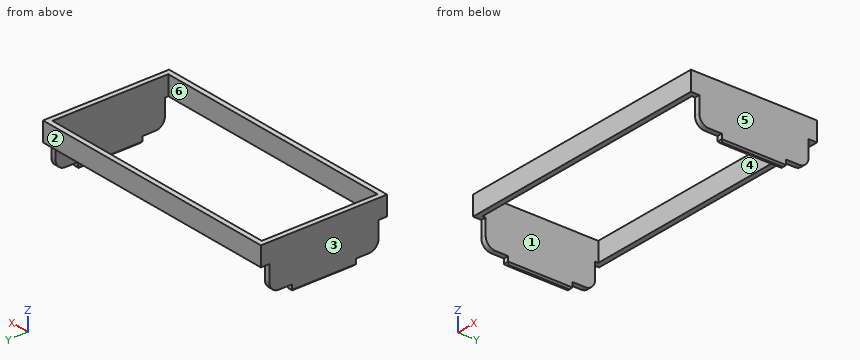
from build123d import *

# Parameters (mm, degrees)
SKETCH1_W           = 80.8
SKETCH1_H           = 39.2
SKETCH1_W_2         = 77.6
SKETCH1_H_2         = 36
BOSS_EXTRUDE1_DEPTH = 6
SKETCH2_W           = 1.6
SKETCH2_H           = 36
BOSS_EXTRUDE2_DEPTH = 8
MOVE_FACE1_BY       = 1
MOVE_FACE1_2_BY     = 1
MOVE_FACE1_3_BY     = 1
MOVE_FACE1_4_BY     = 1
SKETCH3_W           = 1.6
SKETCH3_H           = 20
BOSS_EXTRUDE3_DEPTH = 2
CHAMFER1_SIZE       = 0.5
FILLET1_R           = 3


with BuildPart() as part:
    # Sketch1 → Boss-Extrude1 (new body)
    with BuildSketch(Plane.XY):
        with Locations((38.8, -18)):
            Rectangle(SKETCH1_W, SKETCH1_H)
        with Locations((38.8, -18)):
            Rectangle(SKETCH1_W_2, SKETCH1_H_2, mode=Mode.SUBTRACT)
    extrude(amount=BOSS_EXTRUDE1_DEPTH)

    # Sketch2 → Boss-Extrude2 (add)
    with BuildSketch(Plane(origin=(0, 0, 0), x_dir=(-1, 0, 0), z_dir=(0, 0, -1))):
        with Locations((-78.4, -18)):
            Rectangle(SKETCH2_W, SKETCH2_H)
        with Locations((0.8, -18)):
            Rectangle(SKETCH2_W, SKETCH2_H)
    extrude(amount=BOSS_EXTRUDE2_DEPTH)

    # Move Face1: a face moved inward by 1.0
    extrude(part.faces().sort_by_distance((78.4, 0, -4))[0], amount=MOVE_FACE1_BY, dir=(0, -1, 0), mode=Mode.SUBTRACT)

    # Move Face1 2: a face moved inward by 1.0
    extrude(part.faces().sort_by_distance((78.4, -36, -4))[0], amount=MOVE_FACE1_2_BY, dir=(0, 1, 0), mode=Mode.SUBTRACT)

    # Move Face1 3: a face moved inward by 1.0
    extrude(part.faces().sort_by_distance((-0.8, -36, -4))[0], amount=MOVE_FACE1_3_BY, dir=(0, 1, 0), mode=Mode.SUBTRACT)

    # Move Face1 4: a face moved inward by 1.0
    extrude(part.faces().sort_by_distance((-0.8, 0, -4))[0], amount=MOVE_FACE1_4_BY, dir=(0, -1, 0), mode=Mode.SUBTRACT)

    # Sketch3 → Boss-Extrude3 (add)
    with BuildSketch(Plane(origin=(0, 0, -8), x_dir=(-1, 0, 0), z_dir=(0, 0, -1))):
        with Locations((-78.4, -18)):
            Rectangle(SKETCH3_W, SKETCH3_H)
        with Locations((0.8, -18)):
            Rectangle(SKETCH3_W, SKETCH3_H)
    extrude(amount=BOSS_EXTRUDE3_DEPTH)

    # Chamfer1
    chamfer1_edges = [part.edges().sort_by_distance(p)[0] for p in [
        (78.4, -28, -10),
        (77.6, -18, -10),
        (78.4, -8, -10),
        (79.2, -18, -10),
        (0, -18, -10),
        (-0.8, -28, -10),
        (-1.6, -18, -10),
        (-0.8, -8, -10),
    ]]
    chamfer(chamfer1_edges, length=CHAMFER1_SIZE)

    # Fillet1
    fillet1_edges = [part.edges().sort_by_distance(p)[0] for p in [
        (78.4, -1, -8),
        (78.4, -35, -8),
        (-0.8, -1, -8),
        (-0.8, -35, -8),
    ]]
    fillet(fillet1_edges, radius=FILLET1_R)


solid = part.part
Could you check a few things on this model? Use its own coordinates, in mm. Face numbers are marked on the shaded views. A direction names the side the tool comes from. Give positions to 0.01 mm unless a question says otherwise; leave off trailing zeros. Write each loop counter-clockwise with the first axis right and the second up, starting at its lowest first coordinate (ties: lowest second). Pieces come first, ordered by that corner, then holes. Notation, with made-up numbers: (60, 54) - (79, 54) arc R30 ccw to (79, 81) - close; hole circle Ø2 at (-29.5, -36.75). An arc over 180 degrees is marked (long way). Use CSV: the item, a comma, the result in double quotes. Start each with the question number.
Item 1: For the marked faces 5 and 6, which set-ups out of +Z, -Z, +X, -X, +Y, -Y let a thin tool reach every point of the face, with its end or its side?
Item 2: I want a section at C-C, the plane z = 3.25. Please give me the cut outline in (x, y), then the cut area to 3 significant figures.
Item 3: If we mould it in two halves opening along Y, with no side actions, what happens to the marked faces 1, 2, 3 and 4? For each: pulls with the +Y half, pulls with the -Y half, needs draft (parallel to the pull), parting line crosses it, or undercut.
Item 4: I'm going to push flat-ended pins straight in: pin 1 (6 mm diameter, centred on x = 37.5, z = -4, fed in from -Y); pin 2 (1.3 mm diameter, centred on x = -0.5, z = -2, fed in from -Y); pin 3 (1.3 mm diameter, centred on x = -1, y = -30.5, fed in from -Z); pin 4 (1.6 mm diameter, centred on x = -0.5, z = -8.5, fed in from +Y). Where does each tip first touch, or does it pass through?
Item 5: I want a section at A-A, the plane y = -5.5. Please give me the cut outline in (x, z), then the cut area to 3 significant figures.
Item 6: If I drill on line 1 along X through (y, z) = (-17, -8); line 2 along Y through (x, z) = (15.5, 3.75), over which ranges is the centre line in solid material (lowest first)?
Item 7: I want a section at B-B, the plane z = -1.5. Please give me the cut outline in (x, y), then the cut area to 3 significant figures.
Item 8: I want a section at D-D, the plane y = -20. Please give me the cut outline in (x, z).
Findings:
1,face 5,"+Z, -Z, +X, +Y, -Y"
1,face 6,"+Z, -Z"
2,outline,"(-1.6, -37.6) - (79.2, -37.6) - (79.2, 1.6) - (-1.6, 1.6) - close; hole (0, -36) - (77.6, -36) - (77.6, 0) - (0, 0) - close"
2,area,"374 mm2"
3,face 1,"undercut"
3,face 2,"pulls with the +Y half"
3,face 3,"needs draft"
3,face 4,"undercut"
4,pin 1,"passes through"
4,pin 2,"stops at y = -35"
4,pin 3,"stops at z = -8"
4,pin 4,"stops at y = -2.69"
5,outline,"(-1.6, -8) - (0, -8) - (0, 6) - (-1.6, 6) - close; (77.6, -8) - (79.2, -8) - (79.2, 6) - (77.6, 6) - close"
5,area,"44.8 mm2"
6,line 1,"x = -1.6 to 0, 77.6 to 79.2"
6,line 2,"y = -37.6 to -36, 0 to 1.6"
7,outline,"(-1.6, -35) - (0, -35) - (0, -1) - (-1.6, -1) - close; (77.6, -35) - (79.2, -35) - (79.2, -1) - (77.6, -1) - close"
7,area,"109 mm2"
8,outline,"(-1.6, -9.5) - (-1.1, -10) - (-0.5, -10) - (0, -9.5) - (0, 6) - (-1.6, 6) - close; (77.6, -9.5) - (78.1, -10) - (78.7, -10) - (79.2, -9.5) - (79.2, 6) - (77.6, 6) - close"
